```python
from build123d import *

# Parameters (mm, degrees)
EXTRUDE_1_DEPTH     = 15
SKETCH_5_R          = 2.1
CUT_EXTRUDE_2_DEPTH = 30
SKETCH_6_R          = 2
CUT_EXTRUDE_3_DEPTH = 15


with BuildPart() as part:
    # 草图3 → 凸台-拉伸1 (new body)
    with BuildSketch(Plane(origin=(0, 0, 0), x_dir=(1, 0, 0), z_dir=(0, 1, 0))):
        Polygon((0, 0), (400, 0), (400, 10), (385, 10), (385, 25), (400, 25), (400, 35), (0, 35), (0, 25), (15, 25), (15, 10), (0, 10), align=None)
    extrude(amount=EXTRUDE_1_DEPTH)

    # 草图5 → 切除-拉伸2 (cut)
    with BuildSketch(Plane(origin=(0, 15, 0), x_dir=(1, 0, 0), z_dir=(0, 1, 0))):
        with Locations(Location((152.5, 5, 0), (0, 0, 270))):
            Circle(SKETCH_5_R)
        with Locations(Location((152.5, 30, 0), (0, 0, 270))):
            Circle(SKETCH_5_R)
        with Locations(Location((247.5, 5, 0), (0, 0, 270))):
            Circle(SKETCH_5_R)
        with Locations(Location((247.5, 30, 0), (0, 0, 270))):
            Circle(SKETCH_5_R)
    extrude(amount=-CUT_EXTRUDE_2_DEPTH, mode=Mode.SUBTRACT)

    # 草图6 → 切除-拉伸3 (cut)
    with BuildSketch(Plane(origin=(0, 15, 0), x_dir=(1, 0, 0), z_dir=(0, 1, 0))):
        with Locations(Location((350.5, 5, 0), (0, 0, 270))):
            Circle(SKETCH_6_R)
        with Locations(Location((295.5, 5, 0), (0, 0, 270))):
            Circle(SKETCH_6_R)
        with Locations(Location((350.5, 30, 0), (0, 0, 270))):
            Circle(SKETCH_6_R)
        with Locations(Location((295.5, 30, 0), (0, 0, 270))):
            Circle(SKETCH_6_R)
        with Locations(Location((49.5, 30, 0), (0, 0, 90))):
            Circle(SKETCH_6_R)
        with Locations(Location((104.5, 30, 0), (0, 0, 90))):
            Circle(SKETCH_6_R)
        with Locations(Location((104.5, 5, 0), (0, 0, 90))):
            Circle(SKETCH_6_R)
        with Locations(Location((49.5, 5, 0), (0, 0, 90))):
            Circle(SKETCH_6_R)
    extrude(amount=-CUT_EXTRUDE_3_DEPTH, mode=Mode.SUBTRACT)


solid = part.part
```
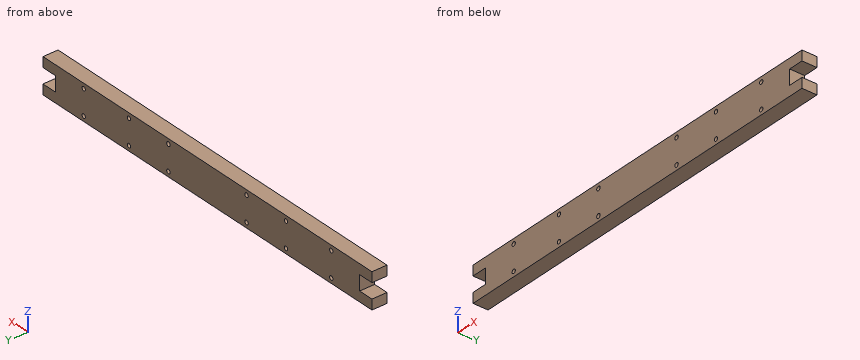
Geometry check sheet. Reference: the model listing, model coordinates, mm. Give positions to 0.01 mm unless a question says otherwise; leave off trailing zeros. Write each loop counter-clockwise with the first axis right and the second up, starting at its lowest first coordinate (ties: lowest second). Pieces come first, ordered by that corner, then holes.
1) Material ranges on L1, parallel to Z at x = 104.5, y = 9.75; L2, parallel to X at y = 11.75, z = -11, recorded low to high.
2) Section check A-A, the plane y = 3.5. State how many separate pieces and enclosed holes the cut face has, and give its area (3 significant figures).
3) Gauge pin test, flat ends, axial feed: pin 1 (2.5 mm diameter, centred on x = 152.5, z = -30, fed in from +Y); pin 2 (7.5 mm diameter, centred on y = 6.5, z = -18, fed in from -X). Record the tip position at first contact, or that the pin passes through.
4) Section check B-B, the plane z = -17. Record the boundary of the cut face in (x, y).
Computed:
1. L1: z = -35 to -32, -28 to -7, -3 to 0
1. L2: x = 15 to 385
2. separate pieces: 1
2. enclosed holes: 12
2. area: 13,400 mm2
3. pin 1: passes through
3. pin 2: stops at x = 15
4. outline: (15, 0) - (385, 0) - (385, 15) - (15, 15) - close
